Model file for the job. Use its own axes, mm. Give positions to 0.01 mm unless a question says otherwise; leave off trailing zeros. Write each loop counter-clockwise with the first axis right and the second up, starting at its lowest first coordinate (ties: lowest second). Pieces come first, ordered by that corner, then holes.
Autodesk Inventor part; units mm, degrees
ref_plane "YZ Plane" through (0, 0, 0) normal (1, 0, 0) x (0, 1, 0)
ref_plane "XZ Plane" through (0, 0, 0) normal (0, 1, 0) x (-1, 0, 0)
ref_plane "XY Plane" through (0, 0, 0) normal (0, 0, 1) x (1, 0, 0)
sketch "Sketch1" plane through (0, 0, 0) normal (0, 1, 0) x (-1, 0, 0)
  line L0 (4.5, 5.5) -> (-7.5, 5.5)
  line L1 (-7.5, 5.5) -> (-7.5, -5.5)
  line L2 (-7.5, -5.5) -> (4.5, -5.5)
  line L3 (4.5, -5.5) -> (4.5, 5.5)
  line L4 (3.5, 3.5) -> (-6.5, 3.5)
  line L5 (-6.5, 3.5) -> (-6.5, -3.5)
  line L6 (-6.5, -3.5) -> (3.5, -3.5)
  line L7 (3.5, -3.5) -> (3.5, 3.5)
  circle A0 centre (1, 4.5) radius 0.375
  circle A1 centre (1, -4.4) radius 0.375
  circle A2 centre (-5, 4.5) radius 0.375
  circle A3 centre (-5, -4.4) radius 0.375
  point P0 (0, 0)
  dimension "d0" = 12
  dimension "d1" = 11
  dimension "d2" = 5.5
  dimension "d3" = 7.5
  dimension "d4" = 10
  dimension "d5" = 7
  dimension "d6" = 2
  dimension "d7" = 1
  dimension "d8" = 0.75
  dimension "d9" = 3.5
  dimension "d10" = 1
  dimension "d13" = 8.9
  dimension "d16" = 6
extrude "Extrusion1" add sketch "Sketch1" along normal blind 1
sketch "Sketch2" plane through (7.5, 0, 5.5) normal (1, 0, 0) x (0, 0, -1)
  circle A0 centre (5.5, -20) radius 20
  line L0 (0, 0) -> (11, 0)
  line L1 (0, 0) -> (0, -0.7711)
  line L2 (11, 0) -> (11, -0.7711)
  arc A1 (11, -0.7711) -> (0, -0.7711) centre (5.5, -20) ccw
  point P0 (5.5, 0)
extrude "Extrusion2" add sketch "Sketch2" against normal up to surface (12 mm away) contours A0 L0 L2 | L1 L0 A0
sketch "Sketch3" plane through (0, 1, 0) normal (0, 1, 0) x (1, 0, 0)
  circle A0 centre (5, 4.4) radius 0.375
  circle A1 centre (5, -4.5) radius 0.375
  circle A2 centre (-1, -4.5) radius 0.375
  circle A3 centre (-1, 4.4) radius 0.375
  line L0 (6.5, 3.5) -> (6.5, -3.5)
  line L1 (-3.5, 3.5) -> (6.5, 3.5)
  line L2 (-3.5, -3.5) -> (-3.5, 3.5)
  line L3 (6.5, -3.5) -> (-3.5, -3.5)
  line L4 (6.5, 3.5) -> (-3.5, 3.5)
  line L5 (-3.5, 3.5) -> (-3.5, -3.5)
  line L6 (-3.5, -3.5) -> (6.5, -3.5)
  line L7 (6.5, -3.5) -> (6.5, 3.5)
  circle A4 centre (5, 4.4) radius 0.375
  circle A5 centre (5, -4.5) radius 0.375
  circle A6 centre (-1, -4.5) radius 0.375
  circle A7 centre (-1, -4.5) radius 0.375
  circle A8 centre (-1, 4.4) radius 0.375
  point P0 (0, 0)
extrude "Extrusion3" cut sketch "Sketch3" against normal through all
properties part number "Eyepiece Mount"
1. Slice it at B-B, the plane z = 0.25. Write the cut outline in (x, y).
Calculated:
outline: (-4.5, 0) - (-3.5, 0) - (-3.5, 1) - (-4.5, 1) - close; (6.5, 0) - (7.5, 0) - (7.5, 1) - (6.5, 1) - close
2. Slice it at A-A, the plane x = 2.5. Write the cut outline in (y, z).
Calculated:
outline: (-0.77, -5.5) - (1, -5.5) - (1, -3.5) - (-0.31, -3.5) arc R20 cw to start; (-0.77, 5.5) arc R20 cw to (-0.31, 3.5) - (1, 3.5) - (1, 5.5) - close
3. Slice it at C-C, the plane x = 5. Write the cut outline in (y, z) (3 decimals), and give its area (3 significant figures).
Calculated:
outline: (-0.771, -5.5) - (1, -5.5) - (1, -4.775) - (-0.578, -4.775) arc R20 cw to start; (-0.771, 5.5) arc R20 cw to (-0.603, 4.875) - (1, 4.875) - (1, 5.5) - close; (-0.43, 4.125) arc R20 cw to (-0.309, 3.5) - (1, 3.5) - (1, 4.125) - close; (-0.409, -4.025) - (1, -4.025) - (1, -3.5) - (-0.309, -3.5) arc R20 cw to start
area: 3.83 mm2
4. Probe probe 1 along X at (y, z) = (-0.35, -4.4) (3 decimals); probe 2 along Z at (x, y) = (5, -0.2) (3 decimals); probe 3 along Z at (x, y) = (1.5, -0.1). List the from-to ranges inside material, lowest first.
Calculated:
probe 1: x = -4.5 to -1.375, -0.625 to 4.625, 5.375 to 7.5
probe 2: z = -5.5 to -4.775, -4.025 to -3.5, 3.5 to 4.125, 4.875 to 5.5
probe 3: z = -5.5 to -3.5, 3.5 to 5.5
5. Pin check, flat tip, straight feed: P1, Ø4, axis at x = 3, z = -1, coming from the +Y side. Stop position of the tip, or through.
Calculated:
P1: passes through
